Source: CAD feature listing. Evaluate the final solid. Frame: model axes, mm. Face numbers are marked on the shaded views. Round coordinates to 2 decimals unless told otherwise and drop trailing zeros. Order: outer loops, then holes, each group sorted by start corner. A loop starts at its lowest first (then second) coordinate and runs counter-clockwise, first axis right, second up. Notation, with made-up numbers: M 46,8 L 77,8 A24 ccw 77,25 Z; hole C 64,60.5 d5. An arc over 180 degrees is marked long. Answer in a Markdown table with one row per item. Add a question column.
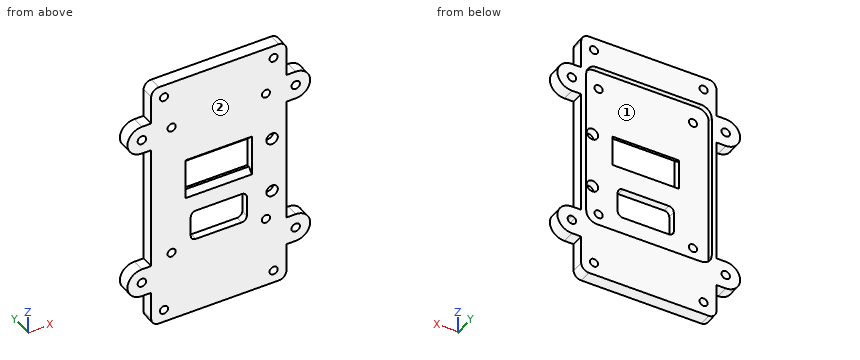
```python
from build123d import *

# Parameters (mm, degrees)
SKETCH1_W           = 47
SKETCH1_H           = 64
BOSS_EXTRUDE1_DEPTH = 5
SKETCH2_W           = 22
SKETCH2_H           = 12
SKETCH2_W_2         = 26
CUT_EXTRUDE1_DEPTH  = 5
SKETCH3_R           = 1.6
CUT_EXTRUDE2_DEPTH  = 63
FILLET1_R           = 2
FILLET2_R           = 3
SKETCH5_R           = 1.65
BOSS_EXTRUDE3_DEPTH = 5
CUT_EXTRUDE5_DEPTH  = 2
SKETCH7_R           = 1.6
CUT_EXTRUDE7_DEPTH  = 66.823356227
CHAMFER4_SIZE       = 2
FILLET3_R           = 3
SKETCH8_R           = 2.25
CUT_EXTRUDE8_DEPTH  = 66.823356227


with BuildPart() as part:
    # Sketch1 → Boss-Extrude1 (new body)
    with BuildSketch(Plane(origin=(0, 0, 0), x_dir=(1, 0, 0), z_dir=(0, 1, 0))):
        Rectangle(SKETCH1_W, SKETCH1_H)
    extrude(amount=BOSS_EXTRUDE1_DEPTH)

    # Sketch2 → Cut-Extrude1 (cut)
    with BuildSketch(Plane(origin=(0, 5, 0), x_dir=(1, 0, 0), z_dir=(0, 1, 0))):
        with Locations((0, 18.81)):
            Rectangle(SKETCH2_W, SKETCH2_H)
        with Locations((0, -2)):
            Rectangle(SKETCH2_W_2, SKETCH2_H)
    extrude(amount=-CUT_EXTRUDE1_DEPTH, mode=Mode.SUBTRACT)

    # Sketch3 → Cut-Extrude2 (cut)
    with BuildSketch(Plane(origin=(0, 5, 0), x_dir=(1, 0, 0), z_dir=(0, 1, 0))):
        with Locations(Location((-18.5, 27, 0), (0, 0, 270))):
            Circle(SKETCH3_R)
        with Locations(Location((18.5, 27, 0), (0, 0, 90))):
            Circle(SKETCH3_R)
        with Locations(Location((-18.5, -26, 0), (0, 0, 270))):
            Circle(SKETCH3_R)
        with Locations(Location((18.5, -26, 0), (0, 0, 90))):
            Circle(SKETCH3_R)
    extrude(amount=-CUT_EXTRUDE2_DEPTH, mode=Mode.SUBTRACT)

    # Fillet1
    fillet1_edges = [part.edges().sort_by_distance(p)[0] for p in [
        (11, 2.5, -12.81),
        (-11, 2.5, -12.81),
        (-11, 2.5, -24.81),
        (11, 2.5, -24.81),
    ]]
    fillet(fillet1_edges, radius=FILLET1_R)

    # Fillet2
    fillet2_edges = [part.edges().sort_by_distance(p)[0] for p in [
        (23.5, 2.5, -32),
        (23.5, 2.5, 32),
        (-23.5, 2.5, 32),
        (-23.5, 2.5, -32),
    ]]
    fillet(fillet2_edges, radius=FILLET2_R)

    # Sketch5 → Boss-Extrude3 (add)
    with BuildSketch(Plane(origin=(0, 5, 0), x_dir=(1, 0, 0), z_dir=(0, 1, 0))):
        with BuildLine():
            ThreePointArc((-30.165, 40.815), (-35.815, 35.165), (-30.165, 29.515))
            Line((-30.165, 29.515), (-26.5, 29.515))
            Line((-26.5, 29.515), (-26.5, -19.515))
            Line((-26.5, -19.515), (-30.165, -19.515))
            ThreePointArc((-30.165, -19.515), (-35.815, -25.165), (-30.165, -30.815))
            Line((-30.165, -30.815), (-26.5, -30.815))
            Line((-26.5, -30.815), (-26.5, -45))
            Line((-26.5, -45), (26.5, -45))
            Line((26.5, -45), (26.5, -30.815))
            Line((26.5, -30.815), (30.165, -30.815))
            ThreePointArc((30.165, -30.815), (35.815, -25.165), (30.165, -19.515))
            Line((30.165, -19.515), (26.5, -19.515))
            Line((26.5, -19.515), (26.5, 29.515))
            Line((26.5, 29.515), (30.165, 29.515))
            ThreePointArc((30.165, 29.515), (35.815, 35.165), (30.165, 40.815))
            Line((30.165, 40.815), (26.5, 40.815))
            Line((26.5, 40.815), (26.5, 55))
            Line((26.5, 55), (-26.5, 55))
            Line((-26.5, 55), (-26.5, 40.815))
            Line((-26.5, 40.815), (-30.165, 40.815))
        make_face()
        with Locations(Location((-30.165, -25.165, 0), (0, 0, 270))):
            Circle(SKETCH5_R, mode=Mode.SUBTRACT)
        with BuildLine():
            ThreePointArc((-20.5, -32), (-22.621320344, -31.121320344), (-23.5, -29))
            Line((-23.5, -29), (-23.5, 29))
            ThreePointArc((-23.5, 29), (-22.621320344, 31.121320344), (-20.5, 32))
            Line((-20.5, 32), (20.5, 32))
            ThreePointArc((20.5, 32), (22.621320344, 31.121320344), (23.5, 29))
            Line((23.5, 29), (23.5, -25.165))
            Line((23.5, -25.165), (23.5, -29))
            ThreePointArc((23.5, -29), (22.621320344, -31.121320344), (20.5, -32))
            Line((20.5, -32), (-20.5, -32))
        make_face(mode=Mode.SUBTRACT)
        with Locations(Location((30.165, -25.165, 0), (0, 0, 270))):
            Circle(SKETCH5_R, mode=Mode.SUBTRACT)
        with Locations(Location((-30.165, 35.165, 0), (0, 0, 270))):
            Circle(SKETCH5_R, mode=Mode.SUBTRACT)
        with BuildLine():
            ThreePointArc((28.998273811, 33.998273811), (30.796427663, 36.689401229), (30.165, 33.515))
            ThreePointArc((30.165, 33.515), (29.533572337, 33.640598771), (28.998273811, 33.998273811))
        make_face(mode=Mode.SUBTRACT)
    extrude(amount=-BOSS_EXTRUDE3_DEPTH)

    # Sketch6 → Cut-Extrude5 (cut)
    with BuildSketch(Plane(origin=(0, 5, 0), x_dir=(1, 0, 0), z_dir=(0, 1, 0))):
        with BuildLine():
            Line((-24.7, 29), (-24.7, -29))
            ThreePointArc((-24.7, -29), (-23.469848481, -31.969848481), (-20.5, -33.2))
            Line((-20.5, -33.2), (20.331389121, -33.2))
            ThreePointArc((20.331389121, -33.2), (23.301237602, -31.969848481), (24.531389121, -29))
            Line((24.531389121, -29), (24.531389121, 29))
            ThreePointArc((24.531389121, 29), (23.301237602, 31.969848481), (20.331389121, 33.2))
            Line((20.331389121, 33.2), (-20.5, 33.2))
            ThreePointArc((-20.5, 33.2), (-23.469848481, 31.969848481), (-24.7, 29))
        make_face()
    extrude(amount=-CUT_EXTRUDE5_DEPTH, mode=Mode.SUBTRACT)

    # Sketch7 → Cut-Extrude7 (cut, through all)
    with BuildSketch(Plane.XZ):
        with Locations(Location((-21.5, 40, 0), (0, 0, 270))):
            Circle(SKETCH7_R)
        with Locations(Location((21.5, 40, 0), (0, 0, 90))):
            Circle(SKETCH7_R)
        with Locations(Location((-21.5, -50, 0), (0, 0, 270))):
            Circle(SKETCH7_R)
        with Locations(Location((21.5, -50, 0), (0, 0, 90))):
            Circle(SKETCH7_R)
    extrude(amount=-CUT_EXTRUDE7_DEPTH, mode=Mode.SUBTRACT)

    # Chamfer4
    chamfer4_edges = [part.edges().sort_by_distance(p)[0] for p in [
        (0, 0, -4),
        (0, 0, 8),
    ]]
    chamfer(chamfer4_edges, length=CHAMFER4_SIZE)

    # Fillet3
    fillet3_edges = [part.edges().sort_by_distance(p)[0] for p in [
        (26.5, 2.5, -55),
        (-26.5, 2.5, -55),
        (-26.5, 2.5, 45),
        (26.5, 2.5, 45),
    ]]
    fillet(fillet3_edges, radius=FILLET3_R)

    # Sketch8 → Cut-Extrude8 (cut, through all)
    with BuildSketch(Plane.XZ):
        with Locations(Location((20.90630532, -16, 0), (0, 0, 270))):
            Circle(SKETCH8_R)
        with Locations(Location((20.90630532, 6, 0), (0, 0, 270))):
            Circle(SKETCH8_R)
    extrude(amount=-CUT_EXTRUDE8_DEPTH, mode=Mode.SUBTRACT)


solid = part.part
```
(1) Pin query (flat end, axial travel): pin 1 (2.5 mm diameter, centred on y = 3, z = 4.5, fed in from +X); pin 2 (4 mm diameter, centred on x = 18.5, z = -27, fed in from +Y); pin 3 (1.5 mm diameter, centred on y = 1, z = -1.5, fed in from -X). Return the tip coordinate at first contact, or that it passes through.
(2) Cut plane C-C (x = 7.5). Return loops of the section in (y, z), and give its area (3 significant figures).
(3) Cut plane A-A (x = -18.5). Return loops of the section in (y, z), and give its area (3 significant figures).
(4) Cut plane B-B (z = -27). Return loops of the section in (x, y), and give its area (3 significant figures).
(5) Draft query along Z for the marked faces 1 and 2. Return one class per face: +Z half, -Z half, draft (parallel to the pull), parting line (faces both ways), or undercut.
(6) Line query: line 1 (X direction, y = 2.4, z = -50); line 2 (Z direction, x = -0.5, y = 2.9); line 3 (Z direction, x = 11.5, y = 3.8). Output: solid intervals per line, ascending. Write a range as from..to.
(7) Cut plane D-D (z = 40). Return loops of the section in (x, y), and give its area (3 significant figures).
Answer list:
| question | item | result |
|---|---|---|
| 1 | pin 1 | x = 26.5 |
| 1 | pin 2 | y = 3 |
| 1 | pin 3 | x = -26.5 |
| 2 | outline | M 0,-55 L 5,-55 L 5,-33.2 L 3,-33.2 L 3,-24.81 L 0,-24.81 Z; M 0,-12.81 L 3,-12.81 L 3,-4 L 2,-4 L 0,-6 Z; M 0,10 L 2,8 L 3,8 L 3,33.2 L 5,33.2 L 5,45 L 0,45 Z |
| 2 | area | 291 mm² |
| 3 | outline | M 0,-55 L 5,-55 L 5,-33.2 L 3,-33.2 L 3,-28.6 L 0,-28.6 Z; M 0,-25.4 L 3,-25.4 L 3,24.4 L 0,24.4 Z; M 0,27.6 L 3,27.6 L 3,33.2 L 5,33.2 L 5,45 L 0,45 Z |
| 3 | area | 348 mm² |
| 4 | outline | M -26.5,0 L -20.1,0 L -20.1,3 L -24.7,3 L -24.7,5 L -26.5,5 Z; M -16.9,0 L 16.9,0 L 16.9,3 L -16.9,3 Z; M 20.1,0 L 26.5,0 L 26.5,5 L 24.53,5 L 24.53,3 L 20.1,3 Z |
| 4 | area | 147 mm² |
| 5 | face 1 | undercut |
| 5 | face 2 | draft |
| 6 | line 1 | -26.5..-23.1, -19.9..19.9, 23.1..26.5 |
| 6 | line 2 | -55..-24.81, -12.81..-4, 8..45 |
| 6 | line 3 | -55..-33.2, 33.2..45 |
| 7 | outline | M -26.5,0 L -23.1,0 L -23.1,5 L -26.5,5 Z; M -19.9,0 L 19.9,0 L 19.9,5 L -19.9,5 Z; M 23.1,0 L 26.5,0 L 26.5,5 L 23.1,5 Z |
| 7 | area | 233 mm² |
